Autodesk Inventor part; units mm, degrees
ref_plane "YZ Plane" through (0, 0, 0) normal (1, 0, 0) x (0, 1, 0)
ref_plane "XZ Plane" through (0, 0, 0) normal (0, 1, 0) x (-1, 0, 0)
ref_plane "XY Plane" through (0, 0, 0) normal (0, 0, 1) x (1, 0, 0)
sketch "Sketch1" plane through (0, 0, 0) normal (0, 0, 1) x (1, 0, 0)
  line L0 (-19.05, 4.7625) -> (19.05, 4.7625)
  line L1 (19.05, 4.7625) -> (19.05, -4.7625)
  line L2 (19.05, -4.7625) -> (-19.05, -4.7625)
  line L3 (-19.05, -4.7625) -> (-19.05, 4.7625)
  point P0 (0, 0)
  point P1 (-19.05, 0)
  point P2 (0, 4.7625)
  dimension "d0" = 38.1
  dimension "d1" = 9.525
extrude "Extrusion1" add sketch "Sketch1" along normal blind 5.207
sketch "Sketch2" plane through (0, 0, 5.207) normal (0, 0, 1) x (1, 0, 0)
  line L0 (-19.05, -4.7625) -> (-19.05, 4.7625)
  point P0 (0, 0)
  point P1 (-10.795, 0)
  dimension "d4" = 8.255
hole "Hole1" at (-10.795, 0, 5.207) direction (0, 0, -1) diameter 6.0071 end through all
sketch "Sketch4" plane through (0, 0, 0) normal (1, 0, 0) x (0, 1, 0)
  circle A0 centre (0, 4.1099) radius 1.778
  point P0 (0, 0)
  dimension "d18" = 3.556
sketch "Sketch8" plane through (0, 0, 0) normal (0, 0, -1) x (-1, 0, 0)
  circle A0 centre (10.795, 0) radius 3.0035
  circle A1 centre (10.795, 0) radius 4.7625 construction
  circle A2 centre (10.795, 0) radius 3.1115
  line L0 (-19.05, 4.7625) -> (-19.05, -4.7625)
  line L1 (19.05, 4.7625) -> (-19.05, 4.7625)
  line L2 (-19.05, -4.7625) -> (19.05, -4.7625)
  line L3 (19.05, -4.7625) -> (19.05, 4.7625)
  line L4 (-19.05, 4.7625) -> (19.05, 4.7625)
  line L5 (19.05, 4.7625) -> (19.05, -4.7625)
  line L6 (19.05, -4.7625) -> (-19.05, -4.7625)
  line L7 (-19.05, -4.7625) -> (-19.05, 4.7625)
  point P0 (17.78, -4.7625)
  point P1 (17.78, 4.7625)
  point P2 (0, 0)
  dimension "d52" = 9.525
  dimension "d53" = 6.223
extrude "Extrusion4" [suppressed]
sketch "Sketch9" plane through (0, 0, 0) normal (0, 0, 1) x (1, 0, 0)
  line L0 (3.429, 0.889) -> (10.541, 0.889)
  line L1 (10.541, 0.889) -> (10.541, -0.889)
  line L2 (10.541, -0.889) -> (3.429, -0.889)
  line L3 (3.429, -0.889) -> (3.429, 0.889)
  line L4 (10.541, 0) -> (3.429, 0) construction
  line L5 (6.985, 0.889) -> (6.985, -0.889) construction
  circle A0 centre (-10.795, 0) radius 3.0035
  point P0 (0, 0)
  dimension "d60" = 7.112
  dimension "d61" = 1.778
  dimension "d130" = 17.78
extrude "Extrusion5" cut sketch "Sketch9" along normal up to next contours L0 L1 L2 L3
sketch "Sketch11" plane through (0, 0, 0) normal (0, 0, 1) x (1, 0, 0)
  line L0 (-26.67, 0) -> (26.67, 0)
  circle A0 centre (-10.795, 0) radius 3.0035
  point P0 (0, 0)
  point P1 (14.224, 0)
  dimension "d131" = 25.019
hole "Hole5" at (14.224, 0, 0) direction (0, 0, 1) diameter 3.5687 end through all counterbore diameter 6.0071 counterbore depth 2.667
sketch "Sketch13" plane through (0, 0, 0) normal (0, 1, 0) x (-1, 0, 0)
  line L0 (-10.541, 0) -> (-10.541, 5.207)
  line L1 (-3.429, 0) -> (-3.429, 5.207)
  line L2 (-10.541, 5.207) -> (-3.429, 5.207) construction
  line L3 (-6.985, 5.207) -> (-6.985, 3.302) construction
  point P0 (0, 0)
  point P1 (-8.89, 0.381)
  point P2 (-1.27, 0.381)
  dimension "d98" = 1.905
hole "Hole6" at (6.985, 0, 3.302) direction (0, -1, 0) diameter 1.6256 end through all
hole "Hole7" at (6.985, 0, 3.302) direction (0, 1, 0) diameter 1.5748 end through all
sketch "Sketch18" plane through (0, 0, 5.207) normal (0, 0, 1) x (1, 0, 0)
  circle A0 centre (-10.795, 0) radius 3.0035
  line L0 (-19.05, -4.7625) -> (-19.05, 4.7625)
  line L1 (-19.05, 0.508) -> (-13.7553, 0.508)
  line L2 (-13.7553, 0.508) -> (-13.7553, -0.508)
  line L3 (-13.7553, -0.508) -> (-19.05, -0.508)
  line L4 (-19.05, -0.508) -> (-19.05, 0.508)
  line L5 (-19.05, 0) -> (-13.7553, 0) construction
  point P0 (0, 0)
  point P1 (-19.05, 0)
  dimension "d132" = 1.016
extrude "Extrusion7" cut sketch "Sketch18" against normal up to next contours L2 A0 | A0 L3 L0 L1 picked at (-13.7681, 0.0567)
sketch "Sketch19" plane through (-19.05, -4.7625, 0) normal (0, -1, 0) x (1, 0, 0)
  line L0 (38.1, 5.207) -> (0, 5.207)
  line L1 (0, 0) -> (0, 5.207)
  line L2 (5.2947, 0) -> (5.2947, 5.207) construction
  line L3 (0, 2.6035) -> (5.2947, 2.6035) construction
  line L4 (2.6474, 2.6035) -> (2.6474, 5.207) construction
  circle A0 centre (2.6474, 2.6035) radius 2.2225 construction
  point P0 (19.05, 0)
  dimension "d136" = 0
  dimension "d137" = 4.445
hole "Hole9" at (-16.4026, -4.7625, 2.6035) direction (0, 1, 0) diameter 2.286 end up to surface counterbore diameter 4.445 counterbore depth 2.286
hole "Hole10" at (-16.4026, 0.508, 2.6035) direction (0, 1, 0) diameter 1.5748 end through all
sketch "Sketch20" plane through (0, 0, 5.207) normal (0, 0, 1) x (1, 0, 0)
  circle A0 centre (14.224, 0) radius 1.7844
  point P0 (0, 0)
hole "Hole11" at (14.224, 0, 5.207) direction (0, 0, -1) diameter 6.223 depth 1.905
chamfer "Chamfer9" distance 1.27 angle 45 3 edges at (19.05, 0, 5.207) (-19.05, 2.6352, 5.207) (-19.05, -2.6353, 5.207)
sketch "Sketch15" plane through (0, 0, 0) normal (1, 0, 0) x (0, 1, 0)
  point P0 (0, 0)
sketch "Sketch16" plane through (0, 0, 5.207) normal (0, 0, 1) x (1, 0, 0)
  circle A0 centre (14.224, 0) radius 1.7844
  line L0 (10.541, 0.889) -> (10.541, -0.889)
  line L1 (10.541, -0.889) -> (3.429, -0.889)
  line L2 (3.429, -0.889) -> (3.429, 0.889)
  line L3 (3.429, 0.889) -> (10.541, 0.889)
  circle A1 centre (-12.7, 0) radius 3.0035
  line L4 (19.05, 4.7625) -> (19.05, -4.7625)
  line L5 (-19.05, 4.7625) -> (19.05, 4.7625)
  line L6 (-19.05, -4.7625) -> (-19.05, 4.7625)
  line L7 (19.05, -4.7625) -> (-19.05, -4.7625)
  point P0 (0, 0)
sketch "Sketch14" plane through (0, 0, 5.207) normal (0, 0, 1) x (1, 0, 0)
  circle A0 centre (6.985, 0) radius 4.1275
  line L0 (10.541, 0.889) -> (10.541, -0.889)
  line L1 (10.541, -0.889) -> (3.429, -0.889)
  line L2 (3.429, -0.889) -> (3.429, 0.889)
  line L3 (3.429, 0.889) -> (10.541, 0.889)
  line L4 (-17.78, 4.7625) -> (17.78, 4.7625)
  line L5 (17.78, -4.7625) -> (-17.78, -4.7625)
  line L6 (6.1976, 0.889) -> (6.1976, 4.7625)
  line L7 (7.7724, 0.889) -> (7.7724, 4.7625)
  line L8 (6.1976, 4.7625) -> (7.7724, 4.7625) construction
  line L9 (6.985, 4.7625) -> (6.985, -4.7625) construction
  line L10 (-13.7553, -0.508) -> (-17.78, -0.508)
  line L11 (-17.78, 0.508) -> (-13.7553, 0.508)
  arc A1 (-13.7553, -0.508) -> (-13.7553, 0.508) centre (-10.795, 0) ccw
  line L12 (17.78, 4.7625) -> (17.78, -4.7625)
  line L13 (-17.78, -4.7625) -> (-17.78, -0.508)
  line L14 (-17.78, 0.508) -> (-17.78, 4.7625)
  point P0 (0, 0)
  dimension "d113" = 8.255
extrude "Extrusion6" [suppressed]
fillet "Fillet4" radius 0.889 4 edges at (10.541, 0.889, 2.6035) (10.541, -0.889, 2.6035) (3.429, 0.889, 2.6035) (3.429, -0.889, 2.6035)
fillet "Fillet5" radius 0.762 4 edges at (-19.05, 4.7625, 1.9685) (-19.05, -4.7625, 1.9685) (19.05, 4.7625, 1.9685) (19.05, -4.7625, 1.9685)
chamfer "Chamfer5" distance 0.254 angle 45 11 edges at (0, 4.7625, 5.207) (0, -4.7625, 5.207) (-19.05, -2.2543, 0) (-18.8268, -4.5393, 0) (0, -4.7625, 0) (18.8268, -4.5393, 0) (19.05, 0, 0) (18.8268, 4.5393, 0) (0, 4.7625, 0) (-18.8268, 4.5393, 0) (-19.05, 2.2542, 0)
sketch "Sketch12" plane through (0, 0, 0) normal (0, 1, 0) x (-1, 0, 0)
  point P0 (0, 0)
chamfer "Chamfer8" distance 0.254 angle 45 3 edges at (-7.7914, 0, 0) (14.224, -3.0035, 0) (-7.7914, 0, 5.207)
properties part number "J002886" material "ALUMINUM, 6061-T651"
Model file for the job. Use its own axes, mm. A direction names the side the tool comes from. Give positions to 0.01 mm unless a question says otherwise; leave off trailing zeros. One line per item, written item: value. Start each with the question number.
Q1. Two-plate mould, pull along Z, no slides. Class faces 1 (the flat face through (7, 0.889, 2)), 2 (the cylindrical face through (6.204, 2.853, 3.405)), 3 (the flat face through (0, 0, 5.207)): +Z half, -Z half, draft (parallel to the pull), parting line (faces both ways), or undercut.
Q2. Probe probe 1 along X at (y, z) = (0, 3); probe 2 along X at (y, z) = (0, 1.55); probe 3 along Y at (x, z) = (14, 4.65). List the from-to ranges inside material, lowest first. Write a range as [from, to].
Q3. Saw through at A-A, the plane y = 2.5. State how many separate pieces and enclosed holes the cut face has, plus the area to 3 significant figures.
Q4. Drop flat-ended pins along their axis: pin 1 Ø4 at (x, y) = (14.224, 0) entering from +Z; pin 2 Ø5 at (x, y) = (-10.795, 0) entering from +Z; pin 3 Ø5 at (x, y) = (14, 0) entering from -Z. Give the stop position or say it passes through.
Q5. 3-axis set-ups, long thin cutter, end or side, ignore diameter. For faces 4 (the cylindrical face through (17.156, -0.651, 1.477)), 5 (the flat face through (7, -0.889, 2)), 6 (the cylindrical face through (-16.7, -1.5, 1.5)), 7 (the flat face through (16, -1, 3.302)): which of +Z, -Z, +X, -X, +Y, -Y reach the whole face in a straight line?
Output values:
1. face 1: draft
1. face 2: undercut
1. face 3: +Z half
2. probe 1: x = [-7.79, 3.43], [10.54, 12.44], [16.01, 19.05]
2. probe 2: x = [-7.79, 3.43], [10.54, 11.22], [17.23, 19.05]
2. probe 3: y = [-4.76, -3.1], [3.1, 4.76]
3. separate pieces: 2
3. enclosed holes: 2
3. area: 159 mm²
4. pin 1: stops at z = 3.3
4. pin 2: passes through
4. pin 3: stops at z = 2.67
5. face 4: -Z
5. face 5: +Z, -Z
5. face 6: -Y
5. face 7: +Z
